```python
from build123d import *

# Parameters (mm, degrees)
F1_DEPTH    = 2
F2_DEPTH    = 0.8
F4_DEPTH    = 2
F5_SIZE     = 1
F6_T1_DEPTH = 18.2300979278


# Not quite as in the source:
# - a fillet or chamfer that OpenCascade refuses, or shapes differently, is made with other operations: its cross-section is extruded or revolved along the edge and cut away or added


with BuildPart() as f1:
    # F0 (on Top) → F1 (new body)
    with BuildSketch(Plane.XY):
        with BuildLine():
            Line((35.175, -3.825), (-39, -3.825))
            Line((-39, -3.825), (-39, -5.825))
            Line((-39, -5.825), (35.175, -5.825))
            ThreePointArc((35.175, -5.825), (39.2938970004, -4.1188970004), (41, 0))
            ThreePointArc((41, 0), (39.2938970004, 4.1188970004), (35.175, 5.825))
            Line((35.175, 5.825), (-39, 5.825))
            Line((-39, 5.825), (-39, 3.825))
            Line((-39, 3.825), (35.175, 3.825))
            ThreePointArc((35.175, 3.825), (37.879683438, 2.704683438), (39, 0))
            ThreePointArc((39, 0), (37.879683438, -2.704683438), (35.175, -3.825))
        make_face()
        with BuildLine():
            Line((-39, 3.825), (-39, -3.825))
            Line((-39, -3.825), (35.175, -3.825))
            ThreePointArc((35.175, -3.825), (37.879683438, -2.704683438), (39, 0))
            ThreePointArc((39, 0), (37.879683438, 2.704683438), (35.175, 3.825))
            Line((35.175, 3.825), (-39, 3.825))
        make_face()
    extrude(amount=F1_DEPTH)

    # F0 (on Top) → F2 (join)
    with BuildSketch(Plane.XY):
        with BuildLine():
            Line((35.175, -3.825), (-39, -3.825))
            Line((-39, -3.825), (-39, -5.825))
            Line((-39, -5.825), (35.175, -5.825))
            ThreePointArc((35.175, -5.825), (39.2938970004, -4.1188970004), (41, 0))
            ThreePointArc((41, 0), (39.2938970004, 4.1188970004), (35.175, 5.825))
            Line((35.175, 5.825), (-39, 5.825))
            Line((-39, 5.825), (-39, 3.825))
            Line((-39, 3.825), (35.175, 3.825))
            ThreePointArc((35.175, 3.825), (37.879683438, 2.704683438), (39, 0))
            ThreePointArc((39, 0), (37.879683438, -2.704683438), (35.175, -3.825))
        make_face()
    extrude(amount=-F2_DEPTH)

    # F3 (on face) → F4 (join)
    with BuildSketch(Plane(origin=(0, 0, -0.8), x_dir=(1, 0, 0), z_dir=(0, 0, -1))):
        with BuildLine():
            Line((-39, 3.825), (-39, -3.825))
            Line((-39, -3.825), (35.175, -3.825))
            ThreePointArc((35.175, -3.825), (39, 0), (35.175, 3.825))
            Line((35.175, 3.825), (-39, 3.825))
        make_face()
        with BuildLine():
            Line((35.175, -3.825), (-39, -3.825))
            Line((-39, -3.825), (-39, -5.825))
            Line((-39, -5.825), (35.175, -5.825))
            ThreePointArc((35.175, -5.825), (41, 0), (35.175, 5.825))
            Line((35.175, 5.825), (-39, 5.825))
            Line((-39, 5.825), (-39, 3.825))
            Line((-39, 3.825), (35.175, 3.825))
            ThreePointArc((35.175, 3.825), (39, 0), (35.175, -3.825))
        make_face()
    extrude(amount=F4_DEPTH)

    # F5
    f5_edges = [f1.edges().sort_by_distance(p)[0] for p in [
        (-1.9125, -5.825, -2.8),
        (-1.9125, -5.825, 2),
    ]]
    chamfer(f5_edges, length=F5_SIZE)

    # F6: chamfer of 3 on 2 edges, made by hand

    # F6_s2 → F6_t1 (cut)
    with BuildSketch(Plane.XY.offset(-9.5150489639)):
        Polygon((-39, -2.825), (-36, -5.825), (-39, -5.825), align=None)
        Polygon((-36, 5.825), (-39, 2.825), (-39, 5.825), align=None)
    extrude(amount=F6_T1_DEPTH, mode=Mode.SUBTRACT)


solid = f1.part
```
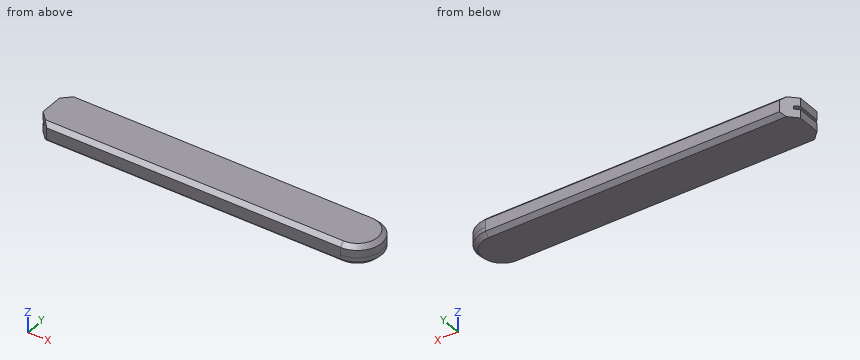
For this review, take the finished solid that the model builds, in its own axes (mm). Round coordinates to 2 decimals unless told otherwise and drop trailing zeros. Write each loop counter-clockwise with the first axis right and the second up, starting at its lowest first coordinate (ties: lowest second). Pieces come first, ordered by that corner, then holes. Notation, with made-up numbers: (72.5, 55) - (101.5, 55) arc R23 cw to (101.5, 68) - close; hole circle Ø11 at (76.25, -38.75). An arc over 180 degrees is marked (long way). Use CSV: the item, a comma, the result in double quotes.
1) Add section A-A on x = -19. Write out the cut boundary in (y, z) (3 decimals).
Conclusion:
outline,"(-5.825, -1.8) - (-4.825, -2.8) - (4.825, -2.8) - (5.825, -1.8) - (5.825, 1) - (4.825, 2) - (-4.825, 2) - (-5.825, 1) - close; hole (-3.825, -0.8) - (3.825, -0.8) - (3.825, 0) - (-3.825, 0) - close"
2) Wall thickness on line 1 along Z through (x, y) = (-23, -0.5); line 2 along Y through (x, z) = (-3, -0.7) (3 decimals); line 3 along Y through (x, z) = (-8, -2.55) (3 decimals): over which ranges is each line inside the solid? List them lowest first. Write a range as from..to.
Conclusion:
line 1,"z = -2.8..-0.8, 0..2"
line 2,"y = -5.825..-3.825, 3.825..5.825"
line 3,"y = -5.075..5.075"
3) Clearance check with a flat-ended pin moving along its axis: pin 1 Ø2 at (y, z) = (-2.5, 1) entering from +X. State where the tip first meets the part, or that it passes through.
Conclusion:
pin 1,"stops at x = 40.8"
